Geometry check sheet. Reference: the model listing, model coordinates, mm. A direction names the side the tool comes from. Coordinates: 2 decimals unless noted, no trailing zeros. Write each loop counter-clockwise with the first axis right and the second up, starting at its lowest first coordinate (ties: lowest second). Pieces come first, ordered by that corner, then holes. Notation, with made-up numbers: (66, 38) -> (86, 38) arc R26 ccw to (86, 77) -> close; hole circle Ø1 at (8, -33). An arc over 180 degrees is marked (long way). Use a Markdown table: item, result.
```python
from build123d import *

# Parameters (mm, degrees)
BOSS_EXTRUDE1_DEPTH = 1.25
FILLET1_R           = 5
FILLET2_R           = 0.5
CUT_EXTRUDE1_DEPTH  = 0.5


with BuildPart() as part:
    # Sketch1 → Boss-Extrude1 (new body, symmetric)
    with BuildSketch(Plane(origin=(0, 0, 0), x_dir=(1, 0, 0), z_dir=(0, 1, 0))):
        with BuildLine():
            Line((6.614378278, 4.5), (65.385621722, 4.5))
            ThreePointArc((65.385621722, 4.5), (80, 0), (65.385621722, -4.5))
            Line((65.385621722, -4.5), (6.614378278, -4.5))
            ThreePointArc((6.614378278, -4.5), (1.506978128, -7.856781588), (-4.479967897, -6.627962556))
            Line((-4.479967897, -6.627962556), (3.5, -2.020725942))
            Line((3.5, -2.020725942), (3.5, 2.020725942))
            Line((3.5, 2.020725942), (0, 4.041451884))
            Line((0, 4.041451884), (-7.979967897, -0.565784729))
            ThreePointArc((-7.979967897, -0.565784729), (-2.623309452, 7.557661511), (6.614378278, 4.5))
        make_face()
        Polygon((72, 4.041451884), (68.5, 2.020725942), (68.5, -2.020725942), (72, -4.041451884), (75.5, -2.020725942), (75.5, 2.020725942), align=None, mode=Mode.SUBTRACT)
    extrude(amount=BOSS_EXTRUDE1_DEPTH, both=True)

    # Fillet1
    fillet1_edges = [part.edges().sort_by_distance(p)[0] for p in [
        (6.614378278, 0, -4.5),
        (65.385621722, 0, -4.5),
        (65.385621722, 0, 4.5),
        (6.614378278, 0, 4.5),
    ]]
    fillet(fillet1_edges, radius=FILLET1_R)

    # Fillet2
    fillet2_edges = [part.edges().sort_by_distance(p)[0] for p in [
        (0.627224524, 1.25, 7.975373935),
        (36, -1.25, -4.5),
        (36, 1.25, -4.5),
        (80, -1.25, 0),
        (80, 1.25, 0),
        (36, -1.25, 4.5),
        (36, 1.25, 4.5),
        (-3.444494595, -1.25, -7.220488694),
        (-3.444494595, 1.25, -7.220488694),
        (64.96037879, -1.25, -4.848697453),
        (64.96037879, 1.25, -4.848697453),
        (64.96037879, -1.25, 4.848697453),
        (64.96037879, 1.25, 4.848697453),
        (7.03962121, -1.25, 4.848697453),
        (7.03962121, 1.25, 4.848697453),
        (7.03962121, -1.25, -4.848697453),
        (7.03962121, 1.25, -4.848697453),
        (0.627224524, -1.25, 7.975373935),
    ]]
    fillet(fillet2_edges, radius=FILLET2_R)

    # Sketch2 → Cut-Extrude1 (cut)
    with BuildSketch(Plane(origin=(0, 1.25, 0), x_dir=(1, 0, 0), z_dir=(0, 1, 0))):
        with BuildLine():
            Line((22, 2.5), (50, 2.5))
            ThreePointArc((50, 2.5), (52.5, 0), (50, -2.5))
            Line((50, -2.5), (22, -2.5))
            ThreePointArc((22, -2.5), (19.5, 0), (22, 2.5))
        make_face()
    cut_extrude1 = extrude(amount=-CUT_EXTRUDE1_DEPTH, mode=Mode.SUBTRACT)

    # Mirror1: Cut-Extrude1 across plane
    add(cut_extrude1.mirror(Plane.ZX), mode=Mode.SUBTRACT)


solid = part.part
```
Item 1: Thickness scan on L1, parallel to Z at x = 58.5, y = 0.15; L2, parallel to X at y = -0.55, z = 0; L3, parallel to Z at x = -2, y = -0.35. Record the ranges inside material, lowest first. Write a range as [from, to].
Answer block:
| item | result |
|---|---|
| L1 | z = [-4.5, 4.5] |
| L2 | x = [-8, -7], [3.5, 68.5], [75.5, 80] |
| L3 | z = [-7.75, -2.89], [5.2, 7.75] |
Item 2: Mould release check, pull along X, two halves, no side actions. Record for faces 1 (the flat face through (37, 1.25, -3)), 2 (the cylindrical face through (64.94, -0.01, 4.84)): +X half, -X half, draft (parallel to the pull), parting line (faces both ways), or undercut.
Answer block:
| item | result |
|---|---|
| face 1 | draft |
| face 2 | undercut |
Item 3: Tool access check on faces 3 (the cylindrical face through (52.5, 1, -0.1)), 4 (the flat face through (-3.934, 0.018, -1.77)), 5 (the cylindrical face through (19.5, -1, 0.1)), 6 (the cylindrical face through (7.015, -0.01, 4.858)), 7 (the flat face through (36, 0, -4.5)). Record the directions out of +Z, -Z, +X, -X, +Y, -Y that give a thin tool (end or side, any length) a straight path to the whole face; none if there is none.
Answer block:
| item | result |
|---|---|
| face 3 | +Y |
| face 4 | +Y, -Y |
| face 5 | -Y |
| face 6 | +Z, +Y, -Y |
| face 7 | -Z, +Y, -Y |
Item 4: Section check A-A on y = -0.35. Record the boundary of the cut face in (x, z), then the cut area to 3 significant figures.
Answer block:
| item | result |
|---|---|
| outline | (-7.98, 0.57) arc R8 ccw to (5.46, -5.85) arc R5 cw to (8.87, -4.5) -> (63.13, -4.5) arc R5 cw to (66.54, -5.85) arc R8 ccw (long way) to (66.54, 5.85) arc R5 cw to (63.13, 4.5) -> (8.87, 4.5) arc R5 cw to (5.46, 5.85) arc R8 ccw to (-4.48, 6.63) -> (3.5, 2.02) -> (3.5, -2.02) -> (0, -4.04) -> close; hole (68.5, -2.02) -> (72, -4.04) -> (75.5, -2.02) -> (75.5, 2.02) -> (72, 4.04) -> (68.5, 2.02) -> close |
| area | 799 mm^2 |
Item 5: Depth check by flat-ended pin: P1, Ø0.8, axis at x = 43, y = 0, coming from the -Z side; P2, Ø1.5, axis at x = 32, z = -1, coming from the +Y side; P3, Ø4, axis at x = 34, z = -1, coming from the +Y side; P4, Ø2.5, axis at x = 28, z = -1, coming from the -Y side. Enter the tip coordinate at first touch or a pass-through.
Answer block:
| item | result |
|---|---|
| P1 | stops at z = -4.5 |
| P2 | stops at y = 0.75 |
| P3 | stops at y = 1.25 |
| P4 | stops at y = -0.75 |
Item 6: Section check B-B on x = 10.5. Record the boundary of the cut face in (y, z), then the cut area to 3 significant figures.
Answer block:
| item | result |
|---|---|
| outline | (-1.25, -4) arc R0.5 ccw to (-0.75, -4.5) -> (0.75, -4.5) arc R0.5 ccw to (1.25, -4) -> (1.25, 4) arc R0.5 ccw to (0.75, 4.5) -> (-0.75, 4.5) arc R0.5 ccw to (-1.25, 4) -> close |
| area | 22.3 mm^2 |
Item 7: Section check C-C on z = -1. Count the separate pieces of the cut face and the enclosed holes in it, then the cut area to 3 significant figures.
Answer block:
| item | result |
|---|---|
| separate pieces | 3 |
| enclosed holes | 0 |
| area | 147 mm^2 |
Item 8: Section check D-D on x = 44. Record the boundary of the cut face in (y, z), then the cut area to 3 significant figures.
Answer block:
| item | result |
|---|---|
| outline | (-1.25, -4) arc R0.5 ccw to (-0.75, -4.5) -> (0.75, -4.5) arc R0.5 ccw to (1.25, -4) -> (1.25, -2.5) -> (0.75, -2.5) -> (0.75, 2.5) -> (1.25, 2.5) -> (1.25, 4) arc R0.5 ccw to (0.75, 4.5) -> (-0.75, 4.5) arc R0.5 ccw to (-1.25, 4) -> (-1.25, 2.5) -> (-0.75, 2.5) -> (-0.75, -2.5) -> (-1.25, -2.5) -> close |
| area | 17.3 mm^2 |
